Verification items for the finished model (mm, model axes). A direction names the side the tool comes from. Give positions to 0.01 mm unless a question says otherwise; leave off trailing zeros. Write each loop counter-clockwise with the first axis right and the second up, starting at its lowest first coordinate (ties: lowest second). Pieces come first, ordered by that corner, then holes. Notation, with made-up numbers: (13, 19) - (50, 19) arc R25 ccw to (50, 42) - close; hole circle Ø2 at (88.5, -17.5). An arc over 180 degrees is marked (long way). Answer as a JSON object with one key per item and string values. Group by question number.
Item 1: Sectioned sample at B-B, the plane x = 55. Record the boundary of the cut face in (y, z).
Item 2: Sectioned sample at C-C, the plane z = -16. Record the boundary of the cut face in (x, y).
Item 3: Sectioned sample at D-D, the plane x = 33. Record the boundary of the cut face in (y, z).
Item 4: Sectioned sample at A-A, the plane y = 31. Record the boundary of the cut face in (x, z).
Item 5: Go/stop test with flat-tipped pins: pin 1 (10 mm diameter, centred on x = 55.5, y = 24.5, fed in from +Z); pin 2 (1.5 mm diameter, centred on y = 34.5, z = -20, fed in from +X); pin 3 (10 mm diameter, centred on x = 50.5, z = -29.5, fed in from +Y). Record where each tip stops, or that it passes through.
Item 6: Scan lines: line 1 along Z through (x, y) = (55, 3); line 2 along Y through (x, z) = (14.5, -3); line 3 along Z through (x, y) = (58, 27). Record each from-to range of solid material in increasing order. Write a range as [from, to].
Item 7: Tool access check on faces 1 (the face through (35, 16, -40)), 2 (the face through (52, 20, -30)), 3 (the face through (35, 5, 0)), 4 (the face through (20, 20, -28)), 5 (the face through (45, 30, -35)). Record the directions out of +Z, -Z, +X, -X, +Y, -Y that give a thin tool (end or side, any length) a straight path to the whole face; none if there is none.
Item 8: Draft check along X on faces 6 (the face through (64.297, 23.986, -35.07)), 7 (the face through (42, 10, -11)), 8 (the face through (30, 30, -28)). Enter one of: +X half, -X half, draft (parallel to the pull), parting line (faces both ways), or undercut.
```python
from build123d import *

# Parameters (mm, degrees)
BOSS_EXTRUDE1_DEPTH            = 40
SKETCH2_W                      = 40
SKETCH2_H                      = 30
BOSS_EXTRUDE2_DEPTH            = 20
BOSS_EXTRUDE3_DEPTH            = 30
CUT_EXTRUDE1_DEPTH             = 30
SKETCH5_W                      = 70
SKETCH5_H                      = 40
BOSS_EXTRUDE4_DEPTH            = 10
SKETCH6_W                      = 20
SKETCH6_H                      = 20
CUT_EXTRUDE2_DEPTH             = 41
F_10_0_10_DIAMETER_HOLE1_D     = 10
F_10_0_10_DIAMETER_HOLE1_DEPTH = 40
FILLET1_R                      = 20


with BuildPart() as part:
    # Sketch1 → Boss-Extrude1 (new body)
    with BuildSketch(Plane(origin=(0, 0, 0), x_dir=(0, -1, 0), z_dir=(-1, 0, 0))):
        Polygon((-10, -12), (-40, -20), (-10, -20), align=None)
    extrude(amount=-BOSS_EXTRUDE1_DEPTH)

    # Sketch2 → Boss-Extrude2 (add)
    with BuildSketch(Plane(origin=(0, 0, -20), x_dir=(-1, 0, 0), z_dir=(0, 0, -1))):
        with Locations((-20, 25)):
            Rectangle(SKETCH2_W, SKETCH2_H)
    extrude(amount=BOSS_EXTRUDE2_DEPTH)

    # Sketch3 → Boss-Extrude3 (add)
    with BuildSketch(Plane(origin=(40, 0, 0), x_dir=(0, 0, -1), z_dir=(1, 0, 0))):
        Polygon((40, 10), (0, 10), (20, 40), (40, 40), align=None)
    extrude(amount=BOSS_EXTRUDE3_DEPTH)

    # Sketch4 → Cut-Extrude1 (cut)
    with BuildSketch(Plane(origin=(70, 0, 0), x_dir=(0, 0, -1), z_dir=(1, 0, 0))):
        Polygon((20, 40), (0, 10), (30, 10), (30, 30), (40, 30), (40, 40), align=None)
    extrude(amount=-CUT_EXTRUDE1_DEPTH, mode=Mode.SUBTRACT)

    # Sketch5 → Boss-Extrude4 (add)
    with BuildSketch(Plane.XZ.offset(-10)):
        with Locations((35, -20)):
            Rectangle(SKETCH5_W, SKETCH5_H)
    extrude(amount=BOSS_EXTRUDE4_DEPTH)

    # Sketch6 → Cut-Extrude2 (cut, through all)
    with BuildSketch(Plane(origin=(0, 0, -40), x_dir=(-1, 0, 0), z_dir=(0, 0, -1))):
        with Locations((-20, 30)):
            Rectangle(SKETCH6_W, SKETCH6_H)
    extrude(amount=-CUT_EXTRUDE2_DEPTH, mode=Mode.SUBTRACT)

    # Ø10.0 (10) Diameter Hole1
    with Locations(Plane(origin=(0, 0, 0), x_dir=(-1, 0, 0), z_dir=(0, -1, 0))):
        with Locations((-55, 15)):
            Hole(F_10_0_10_DIAMETER_HOLE1_D / 2, depth=F_10_0_10_DIAMETER_HOLE1_DEPTH)

    # Fillet1
    fillet1_edges = [part.edges().sort_by_distance(p)[0] for p in [
        (70, 30, -35),
    ]]
    fillet(fillet1_edges, radius=FILLET1_R)


solid = part.part
```
Geometry check:
{
 "1": {"outline": "(0, -40) - (29.36, -40) - (29.36, -30) - (10, -30) - (10, -20) - (0, -20) - close; (0, -10) - (10, -10) - (10, 0) - (0, 0) - close"},
 "2": {"outline": "(0, 0) - (50.1, 0) - (50.1, 10) - (40, 10) - (40, 25) - (30, 25) - (30, 20) - (10, 20) - (10, 25) - (0, 25) - close; (59.9, 0) - (70, 0) - (70, 10) - (59.9, 10) - close"},
 "3": {"outline": "(0, -40) - (40, -40) - (40, -20) - (10, -12) - (10, 0) - (0, 0) - close"},
 "4": {"outline": "(0, -40) - (10, -40) - (10, -17.6) - (0, -17.6) - close; (30, -40) - (40, -40) - (40, -17.6) - (30, -17.6) - close"},
 "5": {"pin 1": "z = -30", "pin 2": "x = 40", "pin 3": "y = 30"},
 "6": {"line 1": "[-40, -20], [-10, 0]", "line 2": "[0, 10]", "line 3": "[-40, -30]"},
 "7": {"face 1": "-Z, +X, -X, +Y, -Y", "face 2": "+Z, +X, +Y", "face 3": "+Z, +X, -X, +Y, -Y", "face 4": "+Z, -Z, +Y", "face 5": "+Z, -Z, +X, +Y"},
 "8": {"face 6": "+X half", "face 7": "draft", "face 8": "undercut"}
}
